from build123d import *

# Parameters (mm, degrees)
BOSS_EXTRUDE1_DEPTH                             = 6.35
SKETCH2_R                                       = 2
SKETCH2_R_2                                     = 32.5
SKETCH2_R_3                                     = 4
SKETCH2_R_4                                     = 2.5
CUT_EXTRUDE1_DEPTH                              = 314.363323476
CHAMFER1_SIZE                                   = 10
CSK_FOR_M4_OVAL_HEAD_MACHINE_SCREW1_D           = 4.8
CSK_FOR_M4_OVAL_HEAD_MACHINE_SCREW1_CSINK_D     = 9.4
CSK_FOR_M4_OVAL_HEAD_MACHINE_SCREW1_CSINK_ANGLE = 90
CSK_FOR_M5_OVAL_HEAD_MACHINE_SCREW1_D           = 5.8
CSK_FOR_M5_OVAL_HEAD_MACHINE_SCREW1_CSINK_D     = 10.4
CSK_FOR_M5_OVAL_HEAD_MACHINE_SCREW1_CSINK_ANGLE = 90


with BuildPart() as part:
    # Sketch1 → Boss-Extrude1 (new body)
    with BuildSketch(Plane(origin=(0, 0, 0), x_dir=(1, 0, 0), z_dir=(0, 1, 0))):
        with BuildLine():
            Line((-45, -219.3), (-38.2, -219.3))
            Line((-38.2, -219.3), (-38.2, -269.3))
            ThreePointArc((-38.2, -269.3), (0, -307.5), (38.2, -269.3))
            Line((38.2, -269.3), (38.2, -219.3))
            Line((38.2, -219.3), (45, -219.3))
            Line((45, -219.3), (45, -39.686269666))
            ThreePointArc((45, -39.686269666), (0, 60), (-45, -39.686269666))
            Line((-45, -39.686269666), (-45, -219.3))
        make_face()
    extrude(amount=BOSS_EXTRUDE1_DEPTH)

    # Sketch2 → Cut-Extrude1 (cut, through all)
    with BuildSketch(Plane(origin=(0, 6.35, 0), x_dir=(1, 0, 0), z_dir=(0, 1, 0))):
        with Locations(Location((0, 53, 0), (0, 0, 270))):
            Circle(SKETCH2_R)
        with Locations(Location((31.152618372, 42.877900702, 0), (0, 0, 270))):
            Circle(SKETCH2_R)
        with Locations(Location((50.405995364, 16.377900702, 0), (0, 0, 270))):
            Circle(SKETCH2_R)
        with Locations(Location((50.405995364, -16.377900702, 0), (0, 0, 270))):
            Circle(SKETCH2_R)
        with Locations(Location((31.152618372, -42.877900702, 0), (0, 0, 270))):
            Circle(SKETCH2_R)
        with Locations(Location((0, -53, 0), (0, 0, 270))):
            Circle(SKETCH2_R)
        with Locations(Location((-31.152618371, -42.877900702, 0), (0, 0, 270))):
            Circle(SKETCH2_R)
        with Locations(Location((-50.405995364, -16.377900702, 0), (0, 0, 270))):
            Circle(SKETCH2_R)
        with Locations(Location((-50.405995364, 16.377900702, 0), (0, 0, 270))):
            Circle(SKETCH2_R)
        with Locations(Location((-31.152618371, 42.877900702, 0), (0, 0, 270))):
            Circle(SKETCH2_R)
        with Locations(Location((0, 0, 0), (0, 0, 270))):
            Circle(SKETCH2_R_2)
        with Locations(Location((0, -269.3, 0), (0, 0, 270))):
            Circle(SKETCH2_R_3)
        with Locations(Location((-40, -169.3, 0), (0, 0, 270))):
            Circle(SKETCH2_R_4)
        with Locations(Location((-40, -49.3, 0), (0, 0, 270))):
            Circle(SKETCH2_R_4)
        with Locations(Location((40, -169.3, 0), (0, 0, 90))):
            Circle(SKETCH2_R_4)
        with Locations(Location((40, -49.3, 0), (0, 0, 90))):
            Circle(SKETCH2_R_4)
        with Locations(Location((0, -89.3, 0), (0, 0, 270))):
            Circle(SKETCH2_R_4)
        with Locations(Location((-20, -149.3, 0), (0, 0, 270))):
            Circle(SKETCH2_R_4)
        with Locations(Location((0, -149.3, 0), (0, 0, 270))):
            Circle(SKETCH2_R_4)
        with Locations(Location((20, -149.3, 0), (0, 0, 270))):
            Circle(SKETCH2_R_4)
        with Locations(Location((-22.943057454, 32.766081772, 0), (0, 0, 270))):
            Circle(SKETCH2_R_4)
        with Locations(Location((22.943057454, 32.766081772, 0), (0, 0, 270))):
            Circle(SKETCH2_R_4)
        with Locations(Location((40, -94.3, 0), (0, 0, 270))):
            Circle(SKETCH2_R_4)
    extrude(amount=-CUT_EXTRUDE1_DEPTH, mode=Mode.SUBTRACT)

    # Chamfer1
    # the kernel refuses this chamfer: 10 mm, written as the material it takes off along each edge
    with BuildSketch(Plane(origin=(45, -25.71682988, 219.3), x_dir=(0.027495876610586282, 0, -0.9996219169112968), z_dir=(0, 1, 0))) as chamfer1_piece_1_section:
        Polygon((CHAMFER1_SIZE * 0.999621916911, CHAMFER1_SIZE * 0.0274958766106), (-CHAMFER1_SIZE * 0.0274958766106, CHAMFER1_SIZE * 0.999621916911), (0, 0), align=None)
    chamfer1_piece_1 = extrude(amount=57.783659759, mode=Mode.PRIVATE)
    chamfer1_piece_1 = split(chamfer1_piece_1, bisect_by=Plane(origin=(38.2, 3.175, 215.680305009), z_dir=(1, 0, 0)), keep=Keep.TOP, mode=Mode.PRIVATE)
    add(chamfer1_piece_1, mode=Mode.SUBTRACT)
    with BuildSketch(Plane(origin=(-45, -25.71682988, 219.3), x_dir=(-0.027495876610586282, 0, -0.9996219169112968), z_dir=(0, 1, 0))) as chamfer1_piece_2_section:
        Polygon((CHAMFER1_SIZE * 0.999621916911, -CHAMFER1_SIZE * 0.0274958766106), (-CHAMFER1_SIZE * 0.0274958766106, -CHAMFER1_SIZE * 0.999621916911), (0, 0), align=None)
    chamfer1_piece_2 = extrude(amount=57.783659759, mode=Mode.PRIVATE)
    chamfer1_piece_2 = split(chamfer1_piece_2, bisect_by=Plane(origin=(-38.2, 3.175, 215.680305009), z_dir=(-1, 0, 0)), keep=Keep.TOP, mode=Mode.PRIVATE)
    add(chamfer1_piece_2, mode=Mode.SUBTRACT)

    # CSK for M4 Oval Head Machine Screw1 (through all)
    with Locations(Plane(origin=(-50.405995364, 6.35, 16.377900702), x_dir=(0, 0, 1), z_dir=(0, 1, 0))):
        with Locations((0, 0), (-32.755801404, 0), (-59.255801404, 19.253376993), (-69.377900702, 50.405995364), (-59.255801404, 81.558613736), (-32.755801404, 100.811990728), (0, 100.811990728), (26.5, 81.558613736), (36.622099298, 50.405995364), (26.5, 19.253376993)):
            CounterSinkHole(CSK_FOR_M4_OVAL_HEAD_MACHINE_SCREW1_D / 2, CSK_FOR_M4_OVAL_HEAD_MACHINE_SCREW1_CSINK_D / 2, counter_sink_angle=CSK_FOR_M4_OVAL_HEAD_MACHINE_SCREW1_CSINK_ANGLE)

    # CSK for M5 Oval Head Machine Screw1 (through all)
    with Locations(Plane(origin=(22.943057454, 0, -32.766081772), x_dir=(0, 0, -1), z_dir=(0, -1, 0))):
        with Locations((0, 0), (0, -45.886114908), (-122.066081772, -22.943057454), (-82.066081772, 17.056942546), (-82.066081772, -62.943057454), (-202.066081772, -62.943057454), (-202.066081772, 17.056942546), (-182.066081772, -2.943057454), (-182.066081772, -22.943057454), (-182.066081772, -42.943057454)):
            CounterSinkHole(CSK_FOR_M5_OVAL_HEAD_MACHINE_SCREW1_D / 2, CSK_FOR_M5_OVAL_HEAD_MACHINE_SCREW1_CSINK_D / 2, counter_sink_angle=CSK_FOR_M5_OVAL_HEAD_MACHINE_SCREW1_CSINK_ANGLE)


solid = part.part
Part model, mm, in its own coordinate system. A direction names the side the tool comes from. Give positions to 0.01 mm unless a question says otherwise; leave off trailing zeros. Write each loop counter-clockwise with the first axis right and the second up, starting at its lowest first coordinate (ties: lowest second). Pieces come first, ordered by that corner, then holes.
1) Two-plate mould, pull along X, no slides. Class faces 1 (the face through (-0.84, 3.13, 307.49)), 2 (the face through (20.1, 4.4, 146.4)), 3 (the face through (-41.6, 3.1, 212.7)), 4 (the face through (-39.87, 2.19, 166.29)): released by +X, released by -X, zero draft, split by the parting line, or undercut.
Resolved:
face 1: split by the parting line
face 2: undercut
face 3: released by -X
face 4: undercut
2) Pin check, flat tips, straight feed: pin 1 (2 mm diameter, centred on x = -37.5, y = 1.5, fed in from -Z); pin 2 (3 mm diameter, centred on y = 2, z = 156.5, fed in from +X); pin 3 (1.5 mm diameter, centred on y = 1.5, z = 12.5, fed in from -X). Stop position of each tip, or through.
Resolved:
pin 1: stops at z = -47.62
pin 2: stops at x = 45
pin 3: stops at x = -58.84
3) Cut at C-C on z = 246. Write the cut outline in (x, y).
Resolved:
outline: (-38.2, 0) - (38.2, 0) - (38.2, 6.35) - (-38.2, 6.35) - close
4) Probe L1, parallel to X at y = 5.5, z = 149.3; L2, parallel to X at y = 5, z = 167; L3, parallel to Z at x = -42, y = 2.5. List the from-to ranges inside material, lowest first.
Resolved:
L1: x = -45 to -22.9, -17.1 to -2.9, 2.9 to 17.1, 22.9 to 45
L2: x = -45 to -41.77, -38.23 to 38.23, 41.77 to 45
L3: z = -42.85 to 47.2, 51.4 to 167.2, 171.4 to 212.3
5) Cut at A-A on z = 0. Write the cut outline in (x, y).
Resolved:
outline: (-60, 0) - (-32.5, 0) - (-32.5, 6.35) - (-60, 6.35) - close; (32.5, 0) - (60, 0) - (60, 6.35) - (32.5, 6.35) - close
6) Cut at B-B on z = 127. Write the cut outline in (x, y), then the cut area to 4 significant figures.
Resolved:
outline: (-45, 0) - (45, 0) - (45, 6.35) - (-45, 6.35) - close
area: 571.5 mm2
7) Which spindle directions (+Z, -Z, +X, -X, +Y, -Y) get a long thin tool onto all of the face, cutting with end or side? Do faces 5 (the face through (38.2, 3, 242)), 6 (the face through (52.896, 4.162, 16.705)), 7 (the face through (-45, 3, 123)). Say none if no direction does.
Resolved:
face 5: +Z, +X, +Y, -Y
face 6: +Y
face 7: +Z, -X, +Y, -Y
